Work out the finished part from the listing and answer in its coordinate system (mm). Face numbers are marked on the shaded views. A direction names the side the tool comes from. Round coordinates to 2 decimals unless told otherwise and drop trailing zeros. Loops run counter-clockwise (first coordinate to the right, second up) from the corner with the lowest first, then second, coordinate; pieces in that order, holes last. Notation, with made-up numbers: M 67.25,14 L 82.25,14 A18 ccw 82.25,25 Z; hole C -25.5,-4 d1. An arc over 180 degrees is marked long. One line per item, written item: value.
```python
from build123d import *

# Parameters (mm, degrees)
SKETCH1_W               = 730
SKETCH1_H               = 150
BASE_FLANGE1_DEPTH      = 2.5
EDGE_FLANGE1_DEPTH      = 730
EDGE_FLANGE1_BEND_DEPTH = 730
SKETCH13_R              = 22.5
CUT_EXTRUDE2_DEPTH      = 10
CUT_EXTRUDE3_DEPTH      = 396.173746598
CUT_EXTRUDE3_DEPTH_BACK = 396.173746598
SKETCH14_W              = 631.337566112
SKETCH14_H              = 273.157514278
CUT_EXTRUDE4_DEPTH      = 396.173746598
CUT_EXTRUDE4_DEPTH_BACK = 396.173746598
CUT_EXTRUDE5_DEPTH      = 408.87885472


# Sheet-metal steps are written as plain solids
with BuildPart() as part:
    # Sketch1 → Base-Flange1 (new body)
    with BuildSketch(Plane(origin=(0, 0, 0), x_dir=(0, 0, -1), z_dir=(1, 0, 0))):
        Rectangle(SKETCH1_W, SKETCH1_H)
    extrude(amount=-BASE_FLANGE1_DEPTH)

    # Edge-Flange1 section (across the edge) → Edge-Flange1 (add)
    with BuildSketch(Plane(origin=(-2.5, 75.2, 365), x_dir=(0, -1, 0), z_dir=(0, 0, -1))):
        with BuildLine():
            Line((-2.5, 0.2), (-2.5, 127.5))
            Line((-2.5, 127.5), (0, 127.5))
            Line((0, 127.5), (0, 0.2))
            ThreePointArc((0, 0.2), (0.058578644, 0.058578644), (0.2, 0))
            Line((0.2, 0), (0.2, -2.5))
            ThreePointArc((0.2, -2.5), (-1.709188309, -1.709188309), (-2.5, 0.2))
        make_face()
    extrude(amount=EDGE_FLANGE1_DEPTH)

    # Edge-Flange1 section 2 (across the edge) → Edge-Flange1 bend (add)
    with BuildSketch(Plane(origin=(-2.5, -75.2, -365), x_dir=(0, 1, 0), z_dir=(0, 0, 1))):
        with BuildLine():
            Line((-2.5, 0.2), (-2.5, 127.5))
            Line((-2.5, 127.5), (0, 127.5))
            Line((0, 127.5), (0, 0.2))
            ThreePointArc((0, 0.2), (0.058578644, 0.058578644), (0.2, 0))
            Line((0.2, 0), (0.2, -2.5))
            ThreePointArc((0.2, -2.5), (-1.709188309, -1.709188309), (-2.5, 0.2))
        make_face()
    extrude(amount=EDGE_FLANGE1_BEND_DEPTH)

    # Sketch13 → Cut-Extrude2 (cut)
    with BuildSketch(Plane(origin=(0, 0, 0), x_dir=(0, 0, -1), z_dir=(1, 0, 0))):
        with Locations((265, 0)):
            Circle(SKETCH13_R)
        with Locations((-290, 0)):
            Circle(SKETCH13_R)
    extrude(amount=-CUT_EXTRUDE2_DEPTH, mode=Mode.SUBTRACT)

    # Sketch14 → Cut-Extrude3 (cut, two sides: drawn at the far end of the back side and taken through both)
    with BuildSketch(Plane(origin=(0, 0, 0), x_dir=(0, 0, -1), z_dir=(1, 0, 0)).offset(-CUT_EXTRUDE3_DEPTH_BACK)):
        with Locations((-126.629311255, -14.019673746)):
            Rectangle(SKETCH14_W, SKETCH14_H)
    extrude(amount=CUT_EXTRUDE3_DEPTH + CUT_EXTRUDE3_DEPTH_BACK, mode=Mode.SUBTRACT)

    # Sketch15 → Cut-Extrude4 (cut, two sides: drawn at the far end of the back side and taken through both)
    with BuildSketch(Plane(origin=(0, 0, 0), x_dir=(0, 0, -1), z_dir=(1, 0, 0)).offset(-CUT_EXTRUDE4_DEPTH_BACK)):
        with BuildLine():
            Line((302.266550641, 80.822052704), (310.532003477, 105.351783703))
            Line((310.532003477, 105.351783703), (400.668447303, 94.566226322))
            Line((400.668447303, 94.566226322), (380.252927975, -108.048173048))
            Line((380.252927975, -108.048173048), (291.286888445, -85.029403714))
            ThreePointArc((291.286888445, -85.029403714), (353.805609642, -5.879089735), (302.266550641, 80.822052704))
        make_face()
    extrude(amount=CUT_EXTRUDE4_DEPTH + CUT_EXTRUDE4_DEPTH_BACK, mode=Mode.SUBTRACT)

    # Sketch17 → Cut-Extrude5 (cut, through all)
    with BuildSketch(Plane(origin=(0, 77.7, 0), x_dir=(1, 0, 0), z_dir=(0, 1, 0))):
        with BuildLine():
            Line((-169.942990536, 157.436912633), (-165.65841416, 335.00880021))
            Line((-165.65841416, 335.00880021), (-74.315703794, 325.146670386))
            ThreePointArc((-74.315703794, 325.146670386), (-69.663025193, 253.273874783), (-78.78147448, 181.830190328))
            Line((-78.78147448, 181.830190328), (-169.942990536, 157.436912633))
        make_face()
    extrude(amount=-CUT_EXTRUDE5_DEPTH, mode=Mode.SUBTRACT)


solid = part.part
```
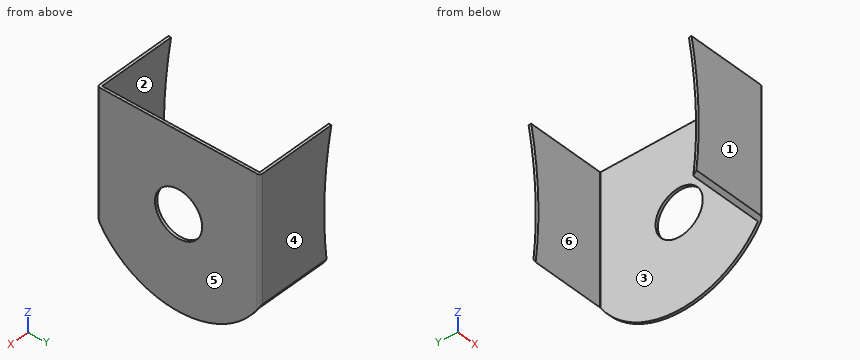
1) Each of these flat-tipped pins is pushed along its axis until it touches: pin 1 (6 mm diameter, centred on y = -47, z = -324, fed in from +X); pin 2 (10 mm diameter, centred on y = -38, z = -209.5, fed in from -X). Where does it stop, or does it pass through?
Check values:
pin 1: x = 0
pin 2: x = -2.5
2) For the marked faces 1 and 2, determine the directions among +Z, -Z, +X, -X, +Y, -Y from which every point of the face is accessible in a straight line to the end or side of a thin tool.
Check values:
face 1: +Z, -Z, +X, -X, -Y
face 2: +Z, -Z, -X
3) Find section D-D (z = -199.5). Give the vertices of the cut face in (x, y).
Check values:
outline: M -75.22,-77.7 L -2.7,-77.7 A2.7 ccw 0,-75 L 0,75 A2.7 ccw -2.7,77.7 L -75.22,77.7 L -75.22,75.2 L -2.7,75.2 A0.2 cw -2.5,75 L -2.5,-75 A0.2 cw -2.7,-75.2 L -75.22,-75.2 Z
4) Find section A-A (y = 0). Give the vertices of the cut face in (x, z).
Check values:
outline: M -2.5,-354 L 0,-354 L 0,-287.5 L -2.5,-287.5 Z; M -2.5,-242.5 L 0,-242.5 L 0,-189.04 L -2.5,-189.04 Z
5) Find the intervals of material crossed by probe 1 along Y at (x, z) = (-35, -294.5); probe 2 along X at (y, z) = (-40, -221.5); probe 3 along Y at (x, z) = (-1.9, -265), in increasing order. Write a range as from..to.
Check values:
probe 1: -77.7..-75.2, 75.2..77.7
probe 2: -2.5..0
probe 3: -77.58..-22.5, 22.5..77.58
6) The mould has two halves that part along Y. Classify the marked faces 3, 4, 5 and 6: +Y half, -Y half, draft (parallel to the pull), parting line (faces both ways), or undercut.
Check values:
face 3: undercut
face 4: +Y half
face 5: draft
face 6: undercut
7) Find section B-B (x = -41). Give the vertices of the cut face in (y, z).
Check values:
outline: M -77.7,-308.4 A89 ccw -75.2,-312.6 L -75.2,-189.04 L -77.7,-189.04 Z; M 75.2,-312.6 A89 ccw 77.7,-308.4 L 77.7,-189.04 L 75.2,-189.04 Z
8) Find section C-C (z = -265). Give the vertices of the cut face in (x, y).
Check values:
outline: M -69.48,-77.7 L -2.7,-77.7 A2.7 ccw 0,-75 L 0,-22.5 L -2.5,-22.5 L -2.5,-75 A0.2 cw -2.7,-75.2 L -69.48,-75.2 Z; M -69.48,75.2 L -2.7,75.2 A0.2 cw -2.5,75 L -2.5,22.5 L 0,22.5 L 0,75 A2.7 ccw -2.7,77.7 L -69.48,77.7 Z
